Input: part model. Units: mm. Frame: model coordinates. A direction names the side the tool comes from. Coordinates: 2 decimals unless noted, no trailing zeros. Write each loop counter-clockwise with the first axis right and the second up, starting at its lowest first coordinate (ties: lowest second). Pieces come first, ordered by that corner, then holes. Notation, with made-up numbers: (-29.5, 61) - (-6.5, 61) arc R30 cw to (-6.5, 96) - close; hole circle Ø10 at (24, 59.5). An arc over 180 degrees is marked (long way). Use a Markdown table: item, result. Add a question column.
Q1. Section query C-C (x = 54). Return the cut outline in (y, z) (3 decimals), then the cut area to 3 significant figures.
Q2. Mould query, pull axis X, two halves, no side actions, for faces 1 (the face through (50.512, 13.078, 33.673)), 2 (the face through (51.75, 0.04, 33.64)), 3 (the face through (15, -5.08, 20)), 4 (the face through (0, -14, 0)). Classes: released by +X, released by -X, zero draft, split by the parting line, or undercut.
Q3. Material intervals for probe 1 along Z at (x, y) = (60, -1) (3 decimals); probe 2 along Y at (x, z) = (50.8, -33.95); probe 3 along Z at (x, y) = (32, -5), sorted ascending. Write a range as from..to.
Q4. Set-up query: faces 5 (the face through (50.512, 13.078, -33.673)), 6 (the face through (14.224, -4, 20)), 7 (the face through (19.4, -16.95, 0.37)), 8 (the face through (48, 0, -32.385)), 9 (the face through (1.651, -4, -20)). Return all of +Z, -Z, +X, -X, +Y, -Y with unobstructed straight access to the full face (end or side cutting, diameter ignored); none if empty.
Q5. Pin query (flat end, axial travel): P1, Ø0.8, axis at x = 14.5, z = -20, coming from the -Y side; P2, Ø8, axis at x = 10.5, z = 19.5, coming from the -Y side; P3, Ø6, axis at x = 28.5, z = 12, coming from the +Y side. Return the tip coordinate at first contact, or that it passes through.
Q6. Section query B-B (y = 7). Return the cut outline in (x, z) (3 decimals), then the cut area to 3 significant figures.
Q7. Section query A-A (z = -23). Return the cut outline in (x, y) (1 decimal).
Q8. Section query D-D (y = -15). Return the cut outline in (x, z) (3 decimals), then the cut area to 3 significant figures.
from build123d import *

# Parameters (mm, degrees)
SKETCH1_R                = 16.9545
BOSS_EXTRUDE1_DEPTH      = 50.8
SKETCH2_R                = 16.9545
BOSS_EXTRUDE2_DEPTH      = 34.925
SKETCH3_R                = 13.081
CUT_EXTRUDE1_DEPTH       = 50.8
SKETCH5_R                = 13.081
CUT_EXTRUDE2_DEPTH       = 69.85
CUT_EXTRUDE4_DEPTH       = 79.088942658
CUT_EXTRUDE4_DEPTH_BACK  = 79.088942658
SKETCH6_R                = 3.81
BOSS_EXTRUDE3_REACH      = 93.464
BOSS_EXTRUDE3_END_RADIUS = 16.9545
SKETCH8_W                = 15.875
SKETCH8_H                = 5.08
CUT_EXTRUDE5_REACH       = 93.464
CUT_EXTRUDE5_END_RADIUS  = 16.9545
SKETCH9_W                = 12.573
SKETCH9_H                = 1.905
SKETCH10_R               = 1.5875
CUT_EXTRUDE6_DEPTH       = 78.461619779
SKETCH11_R               = 13.081
BOSS_EXTRUDE4_DEPTH      = 2.54
SKETCH13_R               = 0.9525
CUT_EXTRUDE8_DEPTH       = 99.778286437


with BuildPart() as part:
    # Sketch1 → Boss-Extrude1 (new body)
    with BuildSketch(Plane(origin=(0, 0, 0), x_dir=(0, 0, -1), z_dir=(1, 0, 0))):
        Circle(SKETCH1_R)
    extrude(amount=BOSS_EXTRUDE1_DEPTH)

    # Sketch2 → Boss-Extrude2 (add, symmetric)
    with BuildSketch(Plane.XY):
        with Locations((50.8, 0)):
            Circle(SKETCH2_R)
    extrude(amount=BOSS_EXTRUDE2_DEPTH, both=True)

    # Sketch3 → Cut-Extrude1 (cut)
    with BuildSketch(Plane.ZY):
        Circle(SKETCH3_R)
    extrude(amount=-CUT_EXTRUDE1_DEPTH, mode=Mode.SUBTRACT)

    # Sketch5 → Cut-Extrude2 (cut)
    with BuildSketch(Plane(origin=(0, 0, -34.925), x_dir=(-1, 0, 0), z_dir=(0, 0, -1))):
        with Locations((-50.8, 0)):
            Circle(SKETCH5_R)
    extrude(amount=-CUT_EXTRUDE2_DEPTH, mode=Mode.SUBTRACT)

    # Sketch6 → Cut-Extrude4 (cut, two sides: drawn at the far end of the back side and taken through both)
    with BuildSketch(Plane(origin=(0, 0, 0), x_dir=(0, 0, -1), z_dir=(1, 0, 0)).offset(-CUT_EXTRUDE4_DEPTH_BACK)):
        with Locations(Location((0, 0, 0), (0, 0, 180))):
            Circle(SKETCH6_R)
    extrude(amount=CUT_EXTRUDE4_DEPTH + CUT_EXTRUDE4_DEPTH_BACK, mode=Mode.SUBTRACT)

    # SurfaceCut1
    split(bisect_by=Plane(origin=(0, 0, 0), x_dir=(1, 0, 0), z_dir=(0, 1, 0)), keep=Keep.BOTTOM)


with BuildPart() as body_2:
    # Boss-Extrude3: up to this cylinder (the profile starts outside it)
    boss_extrude3_end = Plane(origin=(7.9375, 0, 0), z_dir=(-1, 0, 0)) * Cylinder(BOSS_EXTRUDE3_END_RADIUS, 221.837, mode=Mode.PRIVATE)
    # Sketch8 → Boss-Extrude3 (new, up to the surface)
    with BuildSketch(Plane.XY.offset(24.13), mode=Mode.PRIVATE) as boss_extrude3_sk1:
        with Locations((7.9375, -2.54)):
            Rectangle(SKETCH8_W, SKETCH8_H)
    boss_extrude3_tool1 = extrude(boss_extrude3_sk1.sketch, amount=-BOSS_EXTRUDE3_REACH, mode=Mode.PRIVATE) - boss_extrude3_end
    add(boss_extrude3_tool1.solids().sort_by_distance((7.9375, -2.54, 24.13))[0])

    # Cut-Extrude5: up to this cylinder (the profile starts outside it)
    cut_extrude5_end = Plane(origin=(7.9375, 0, 0), z_dir=(-1, 0, 0)) * Cylinder(CUT_EXTRUDE5_END_RADIUS, 221.837, mode=Mode.PRIVATE)
    # Sketch9 → Cut-Extrude5 (cut, up to the surface)
    with BuildSketch(Plane.XY.offset(24.13), mode=Mode.PRIVATE) as cut_extrude5_sk1:
        with Locations((7.9375, -4.1275)):
            Rectangle(SKETCH9_W, SKETCH9_H)
    cut_extrude5_tool1 = extrude(cut_extrude5_sk1.sketch, amount=-CUT_EXTRUDE5_REACH, mode=Mode.PRIVATE) - cut_extrude5_end
    add(cut_extrude5_tool1.solids().sort_by_distance((7.9375, -4.1275, 24.13))[0], mode=Mode.SUBTRACT)


with BuildPart() as body_3:
    # Mirror1: mirrored copy
    add(body_2.part.mirror(Plane.XY))


with BuildPart() as part_1:
    add(part.part)

    # Intersect1: read off the stored shape, not the designer's step
    # Intersect1: union body 3, body 2
    add(body_3.part)
    add(body_2.part)

    # Sketch10 → Cut-Extrude6 (cut, through all)
    with BuildSketch(Plane.XZ.offset(3.175)):
        with Locations(Location((7.9375, 20.392281148, 0), (0, 0, 270))):
            Circle(SKETCH10_R)
    cut_extrude6 = extrude(amount=-CUT_EXTRUDE6_DEPTH, mode=Mode.SUBTRACT)

    # Mirror2: Cut-Extrude6 across plane
    add(cut_extrude6.mirror(Plane.XY), mode=Mode.SUBTRACT)

    # Sketch11 → Boss-Extrude4 (add)
    with BuildSketch(Plane(origin=(0, 0, -34.925), x_dir=(-1, 0, 0), z_dir=(0, 0, -1))):
        with Locations((-50.8, 0)):
            Circle(SKETCH11_R)
    boss_extrude4 = extrude(amount=-BOSS_EXTRUDE4_DEPTH)

    # Mirror3: Boss-Extrude4 across plane
    add(boss_extrude4.mirror(Plane.XY))

    # Sketch13 → Cut-Extrude8 (cut, through all)
    with BuildSketch(Plane(origin=(0, 0, -34.925), x_dir=(-1, 0, 0), z_dir=(0, 0, -1))):
        with Locations((-50.8, 0)):
            Circle(SKETCH13_R)
    extrude(amount=-CUT_EXTRUDE8_DEPTH, mode=Mode.SUBTRACT)


solid = part_1.part
Values follow:
| question | item | result |
|---|---|---|
| 1 | outline | (-16.65, -34.925) - (12.684, -34.925) - (12.684, -32.385) - (-12.684, -32.385) - (-12.684, 32.385) - (12.684, 32.385) - (12.684, 34.925) - (-16.65, 34.925) - close |
| 1 | area | 406 mm2 |
| 2 | face 1 | split by the parting line |
| 2 | face 2 | undercut |
| 2 | face 3 | zero draft |
| 2 | face 4 | released by -X |
| 3 | probe 1 | -34.925..-32.385, 32.385..34.925 |
| 3 | probe 2 | -16.95..-0.95, 0.95..13.08 |
| 3 | probe 3 | -16.2..-12.09, 12.09..16.2 |
| 4 | face 5 | +Z, -Z, +Y |
| 4 | face 6 | +Z, -Y |
| 4 | face 7 | -Y |
| 4 | face 8 | +Y |
| 4 | face 9 | -Z, -Y |
| 5 | P1 | y = -5.08 |
| 5 | P2 | y = -6.87 |
| 5 | P3 | y = 0 |
| 6 | outline | (39.75, -34.925) - (61.85, -34.925) - (61.85, -32.385) - (39.75, -32.385) - close; (39.75, 32.385) - (61.85, 32.385) - (61.85, 34.925) - (39.75, 34.925) - close |
| 6 | area | 112 mm2 |
| 7 | outline | (0, -5.1) - (1.7, -5.1) - (1.7, -3.2) - (14.2, -3.2) - (14.2, -5.1) - (15.9, -5.1) - (15.9, 0) - (0, 0) - close; (33.8, 0) arc R17 ccw to (67.8, 0) - (63.9, 0) arc R13.1 cw to (37.7, 0) - close |
| 8 | outline | (0, -7.903) - (42.897, -7.903) - (42.897, -34.925) - (58.703, -34.925) - (58.703, 34.925) - (42.897, 34.925) - (42.897, 7.903) - (0, 7.903) - close |
| 8 | area | 1,780 mm2 |
